Can you work these out from the drawing? Everything is in mm from the part's minimum corner. A direction names the side the tool comes from. Round coordinates to 2 decimals unless told otherwise and drop trailing zeros. Loops run counter-clockwise (first coordinate to the right, second up) from the corner with the lowest first, then second, coordinate; pieces in that order, holes last. Notation, with made-up numbers: (-17.75, 67.25) -> (-7.75, 67.25) arc R24 ccw to (-7.75, 83.25) -> close; hole circle Ø9 at (10.25, 15.5). An arc over 180 degrees is marked (long way). Answer as a JSON object with one key per item and string values.
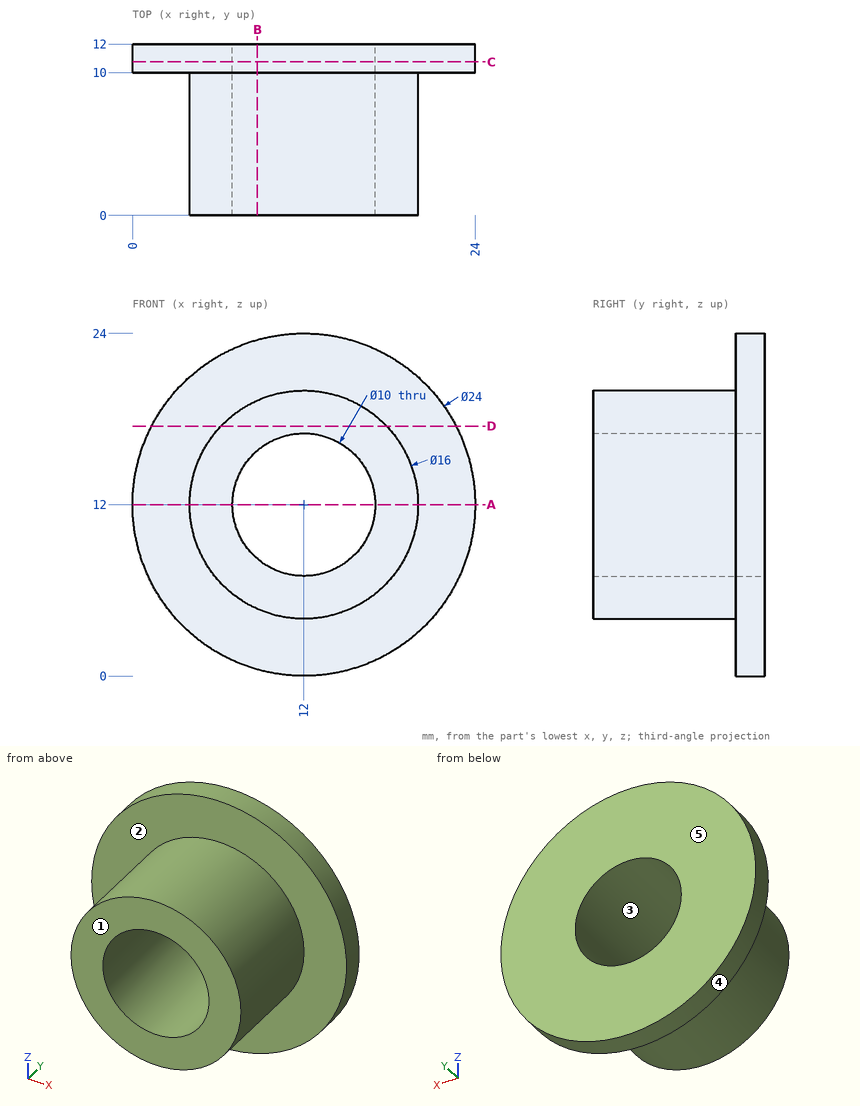
Q1. I want a section at B-B, the plane x = 8.75. Write out the boundary of the cut face in (y, z), then the cut area to 3 significant figures.
Determined:
{"outline": "(0, 4.69) -> (10, 4.69) -> (10, 0.45) -> (12, 0.45) -> (12, 8.2) -> (0, 8.2) -> close; (0, 15.8) -> (12, 15.8) -> (12, 23.55) -> (10, 23.55) -> (10, 19.31) -> (0, 19.31) -> close", "area": "101 mm²"}
Q2. I want a section at D-D, the plane z = 17.5. Write out the boundary of the cut face in (x, y).
Determined:
{"outline": "(1.33, 10) -> (6.19, 10) -> (6.19, 0) -> (17.81, 0) -> (17.81, 10) -> (22.67, 10) -> (22.67, 12) -> (1.33, 12) -> close"}
Q3. I'm going to push flat-ended pins straight in: pin 1 (1 mm diameter, centred on y = 8.5, z = 13.5, fed in from +X); pin 2 (1.5 mm diameter, centred on y = 7, z = 3, fed in from +X); pin 3 (5 mm diameter, centred on y = 9, z = 21.5, fed in from -X); pin 4 (4 mm diameter, centred on y = 7, z = 11, fed in from +X). Where does each tip first touch, or does it pass through?
Determined:
{"pin 1": "x = 19.94", "pin 2": "through", "pin 3": "x = 2.41", "pin 4": "x = 20"}
Q4. On a 3-axis mill with a long thin cutter (end or side, diameter ignored), from which of +Z, -Z, +X, -X, +Y, -Y can I reach the whole of each face in a straight line? I mean the marked faces 1 and 2. Say none if no direction works.
Determined:
{"face 1": "+Z, -Z, +X, -X, -Y", "face 2": "-Y"}
Q5. We'd pull the mould along Z, two halves only. Please class the marked faces 3, 4 and 5: pulls with the +Z half, pulls with the -Z half, needs draft (parallel to the pull), parting line crosses it, or undercut.
Determined:
{"face 3": "undercut", "face 4": "parting line crosses it", "face 5": "needs draft"}
Q6. I want a section at C-C, the plane y = 10.75. Write out the boundary of the cut face in (x, z), then the cut area to 3 significant figures.
Determined:
{"outline": "circle Ø24 at (12, 12); hole circle Ø10 at (12, 12)", "area": "374 mm²"}
Q7. I want a section at A-A, the plane z = 12. Write out the boundary of the cut face in (x, y).
Determined:
{"outline": "(0, 10) -> (4, 10) -> (4, 0) -> (7, 0) -> (7, 12) -> (0, 12) -> close; (17, 0) -> (20, 0) -> (20, 10) -> (24, 10) -> (24, 12) -> (17, 12) -> close"}
Q8. If I drill on L1, parallel to Z at x = 12, y = 5.5; L2, parallel to Z at x = 12.25, y = 10.5; L3, parallel to Y at x = 22, z = 5.5, over which ranges is the centre line in solid material (lowest first)? Write a range as [from, to].
Determined:
{"L1": "[4, 7], [17, 20]", "L2": "[0, 7.01], [16.99, 24]", "L3": "[10, 12]"}
